Can you work these out from the model? Positions are in its coordinate system, mm. Face numbers are marked on the shaded views. A direction names the side the tool comes from. Coordinates: 2 decimals unless noted, no trailing zeros. Order: outer loops, then holes, each group sorted by start corner. A loop starts at its lowest first (then second) coordinate and runs counter-clockwise, first axis right, second up.
```python
from build123d import *

# Parameters (mm, degrees)
SKETCH_1_R      = 2.1
SKETCH_1_R_2    = 4
EXTRUDE_1_DEPTH = 4
EXTRUDE_2_DEPTH = 10.3
EXTRUDE_START   = -14.3
SKETCH_1_6_R    = 2.1
SKETCH_1_6_R_2  = 2.2
EXTRUDE_3_DEPTH = 4
EXTRUDE_4_DEPTH = 6.8
FILLET_1_R      = 5


with BuildPart() as part:
    # 草图1 → 凸台-拉伸1 (new body)
    with BuildSketch(Plane.XY):
        with BuildLine():
            ThreePointArc((-43, 28), (-47.949747468, 25.949747468), (-50, 21))
            Line((-50, 21), (-50, -21))
            ThreePointArc((-50, -21), (-47.949747468, -25.949747468), (-43, -28))
            Line((-43, -28), (-28.5, -28))
            Line((-28.5, -28), (-28.5, 28))
            Line((-28.5, 28), (-43, 28))
        make_face()
        with Locations((-43, 21)):
            Circle(SKETCH_1_R, mode=Mode.SUBTRACT)
        with Locations((-35, 0)):
            Circle(SKETCH_1_R_2, mode=Mode.SUBTRACT)
        with Locations((-43, -21)):
            Circle(SKETCH_1_R, mode=Mode.SUBTRACT)
    extrude(amount=EXTRUDE_1_DEPTH)

    # 草图1<5> → 凸台-拉伸2 (add)
    with BuildSketch(Plane.XY):
        with BuildLine():
            Line((-43, 12.1), (-50, 12.1))
            Line((-50, 12.1), (-50, 10.5))
            Line((-50, 10.5), (-28.5, 10.5))
            Line((-28.5, 10.5), (-28.5, 28))
            Line((-28.5, 28), (-31.5, 28))
            Line((-31.5, 28), (-34.502137832, 18.354940724))
            ThreePointArc((-34.502137832, 18.354940724), (-37.724160141, 13.832328567), (-43, 12.1))
        make_face()
        with BuildLine():
            Line((-28.5, -10.5), (-50, -10.5))
            Line((-50, -10.5), (-50, -12.1))
            Line((-50, -12.1), (-43, -12.1))
            ThreePointArc((-43, -12.1), (-37.724160141, -13.832328567), (-34.502137832, -18.354940724))
            Line((-34.502137832, -18.354940724), (-31.5, -28))
            Line((-31.5, -28), (-28.5, -28))
            Line((-28.5, -28), (-28.5, -10.5))
        make_face()
    extrude(amount=-EXTRUDE_2_DEPTH)

    # 草图1<6> → 凸台-拉伸3 (add)
    with BuildSketch(Plane.XY.offset(EXTRUDE_START)):
        with BuildLine():
            ThreePointArc((-43, 28), (-47.949747468, 25.949747468), (-50, 21))
            Line((-50, 21), (-50, -21))
            ThreePointArc((-50, -21), (-47.949747468, -25.949747468), (-43, -28))
            Line((-43, -28), (-28.5, -28))
            Line((-28.5, -28), (-28.5, 28))
            Line((-28.5, 28), (-43, 28))
        make_face()
        with Locations((-43, 21)):
            Circle(SKETCH_1_6_R, mode=Mode.SUBTRACT)
        with Locations((-43, -21)):
            Circle(SKETCH_1_6_R, mode=Mode.SUBTRACT)
        with Locations((-35, 0)):
            Circle(SKETCH_1_6_R_2, mode=Mode.SUBTRACT)
    extrude(amount=EXTRUDE_3_DEPTH)

    # 草图1<7> → 凸台-拉伸4 (add)
    with BuildSketch(Plane.XY.offset(EXTRUDE_START)):
        with BuildLine():
            Line((-43, 12.1), (-50, 12.1))
            Line((-50, 12.1), (-50, 10.5))
            Line((-50, 10.5), (-28.5, 10.5))
            Line((-28.5, 10.5), (-28.5, 13.5))
            Line((-28.5, 13.5), (-42.118030123, 12.143808429))
            ThreePointArc((-42.118030123, 12.143808429), (-42.558471393, 12.110958854), (-43, 12.1))
        make_face()
        with BuildLine():
            Line((-28.5, -10.5), (-50, -10.5))
            Line((-50, -10.5), (-50, -12.1))
            Line((-50, -12.1), (-43, -12.1))
            ThreePointArc((-43, -12.1), (-42.558471393, -12.110958854), (-42.118030123, -12.143808429))
            Line((-42.118030123, -12.143808429), (-28.5, -13.5))
            Line((-28.5, -13.5), (-28.5, -10.5))
        make_face()
    extrude(amount=-EXTRUDE_4_DEPTH)

    # 圆角1
    fillet_1_edges = [part.edges().sort_by_distance(p)[0] for p in [
        (-50, 11.3, -21.1),
        (-50, -11.3, -21.1),
    ]]
    fillet(fillet_1_edges, radius=FILLET_1_R)


solid = part.part
```
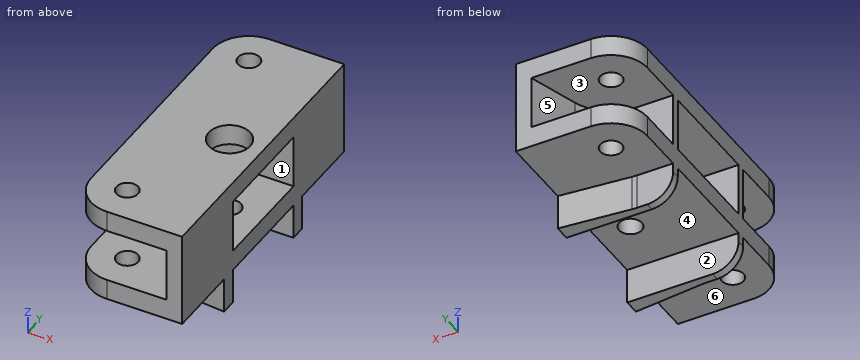
1. Imagine slicing it at B-B on y = -6.5. Please give me the cut outline in (x, z), then the cut area to 3 significant figures.
Completed:
outline: (-50, -14.3) - (-28.5, -14.3) - (-28.5, -10.3) - (-50, -10.3) - close; (-50, 0) - (-28.5, 0) - (-28.5, 4) - (-50, 4) - close
area: 172 mm2
2. Please list where these lines run through material, in increasing order: probe 1 along Y at (x, z) = (-43, 2.45); probe 2 along Z at (x, y) = (-45.5, -16); probe 3 along Y at (x, z) = (-43.5, -3.25).
Completed:
probe 1: y = -28 to -23.1, -18.9 to 18.9, 23.1 to 28
probe 2: z = -14.3 to -10.3, 0 to 4
probe 3: y = -12.1 to -10.5, 10.5 to 12.1
3. On a 3-axis mill with a long thin cutter (end or side, diameter ignored), from which of +Z, -Z, +X, -X, +Y, -Y can I reach the whole of each face in a straight line? I mean the marked faces 1, 2 and 3. Say none if no direction works.
Completed:
face 1: +X, -X
face 2: -Z, +X, -X
face 3: -X, +Y
4. Imagine slicing it at D-D on z = -12.5. Please give me the cut outline in (x, y).
Completed:
outline: (-50, -21) arc R7 ccw to (-43, -28) - (-28.5, -28) - (-28.5, 28) - (-43, 28) arc R7 ccw to (-50, 21) - close; hole circle Ø4.2 at (-43, -21); hole circle Ø4.2 at (-43, 21); hole circle Ø4.4 at (-35, 0)
5. Imagine slicing it at A-A on z = -1.75. Please give me the cut outline in (x, y).
Completed:
outline: (-50, -12.1) - (-43, -12.1) arc R8.9 cw to (-34.5, -18.35) - (-31.5, -28) - (-28.5, -28) - (-28.5, -10.5) - (-50, -10.5) - close; (-50, 10.5) - (-28.5, 10.5) - (-28.5, 28) - (-31.5, 28) - (-34.5, 18.35) arc R8.9 cw to (-43, 12.1) - (-50, 12.1) - close
6. Thinking about a two-plate mould opening in Y: for the marked faces 4, 5 and 6, which applies, pulls with the +Y half, pulls with the -Y half, needs draft (parallel to the pull), parting line crosses it, or undercut?
Completed:
face 4: undercut
face 5: pulls with the +Y half
face 6: needs draft
7. I'm going to push flat-ended pins straight in: pin 1 (8 mm diameter, centred on x = -38, y = -23, fed in from -Z); pin 2 (5.5 mm diameter, centred on x = -47, z = -19.5, fed in from -Y); pin 3 (2 mm diameter, centred on x = -36, z = -18, fed in from -Y); pin 4 (3 mm diameter, centred on y = 16.5, z = -18, fed in from -X). Where does each tip first touch, or does it pass through?
Completed:
pin 1: stops at z = -14.3
pin 2: stops at y = -12.1
pin 3: stops at y = -12.85
pin 4: passes through
8. Imagine slicing it at C-C on y = 0. Please give me the cut outline in (x, z), then the cut area to 3 significant figures.
Completed:
outline: (-50, -14.3) - (-37.2, -14.3) - (-37.2, -10.3) - (-50, -10.3) - close; (-50, 0) - (-39, 0) - (-39, 4) - (-50, 4) - close; (-32.8, -14.3) - (-28.5, -14.3) - (-28.5, -10.3) - (-32.8, -10.3) - close; (-31, 0) - (-28.5, 0) - (-28.5, 4) - (-31, 4) - close
area: 122 mm2
